Build history of the part. All positions in model axes, mm. A direction names the side the tool comes from. Give positions to 0.01 mm unless a question says otherwise; leave off trailing zeros. Write each loop counter-clockwise with the first axis right and the second up, starting at its lowest first coordinate (ties: lowest second). Pieces come first, ordered by that corner, then holes.
from build123d import *

# Parameters (mm, degrees)
BASEHEAD_DEPTH = 4
SKETCH5_R      = 3
BASEBODY_DEPTH = 30
CHAMFER1_SIZE  = 0.3
SCALE_1_SCALE  = 0.25


with BuildPart() as part:
    # Sketch2 → BaseHead (new body)
    with BuildSketch(Plane(origin=(0, 0, 0), x_dir=(0, 0, -1), z_dir=(1, 0, 0))):
        Polygon((0, -5.773502692), (5, -2.886751346), (5, 2.886751346), (0, 5.773502692), (-5, 2.886751346), (-5, -2.886751346), align=None)
    extrude(amount=BASEHEAD_DEPTH)

    # Sketch3 → BearingFace (revolve, cut)
    with BuildSketch(Plane.XY, mode=Mode.PRIVATE) as bearingface_sk:
        Polygon((4, 5.773502692), (4, 4.37), (3.5, 4.87), (3.5, 5.773502692), align=None)
    revolve(bearingface_sk.sketch.rotate(Axis((-0.957090588, 0, 0), (1, 0, 0)), 90), axis=Axis((-0.957090588, 0, 0), (1, 0, 0)), mode=Mode.SUBTRACT)

    # Sketch4 → HeadChamfer (revolve, cut)
    with BuildSketch(Plane.XY):
        Polygon((0, 5.773502692), (0.281531956, 5.773502692), (0, 5), align=None)
    revolve(axis=Axis((-0.493528746, 0, 0), (1, 0, 0)), mode=Mode.SUBTRACT)

    # Sketch5 → BaseBody (add)
    with BuildSketch(Plane(origin=(4, 0, 0), x_dir=(0, 0, -1), z_dir=(1, 0, 0))):
        with Locations(Location((0, 0, 0), (0, 0, 180))):
            Circle(SKETCH5_R)
    extrude(amount=BASEBODY_DEPTH)

    # Chamfer1
    chamfer1_edges = [part.edges().sort_by_distance(p)[0] for p in [
        (34, 0, -3),
    ]]
    chamfer(chamfer1_edges, length=CHAMFER1_SIZE)


with BuildPart() as part_1:
    # 缩放比例1: scaled about (0, 0, 0)
    add(part.part.scale(SCALE_1_SCALE))


solid = part_1.part
(1) Drop a flat-ended pin along its axis: pin 1 (1.5 mm diameter, centred on x = 3, z = 0, fed in from -Y). Give the stop position or say it passes through.
(2) Saw through at B-B, the plane x = 5. List the corners of the cut face in (y, z).
(3) Saw through at A-A, the plane x = 0.5. List the corners of the cut face in (y, z).
(4) Probe line 1 (Z direction, x = 4.5, y = 0.2); line 2 (X direction, y = -0.2, z = -0.9). List the from-to ranges inside material, lowest first.
(5) 3-axis set-ups, long thin cutter, end or side, ignore diameter. For faces 1 (the face through (4.661, -0.225, 0.715)), 2 (the face through (0.4, 0, 1.25)): which of +Z, -Z, +X, -X, +Y, -Y reach the whole face in a straight line?
Computed values:
1. pin 1: stops at y = -0.75
2. outline: circle Ø1.5 at (0, 0)
3. outline: (-1.44, 0) - (-0.72, -1.25) - (0.72, -1.25) - (1.44, 0) - (0.72, 1.25) - (-0.72, 1.25) - close
4. line 1: z = -0.72 to 0.72
4. line 2: x = 0 to 1
5. face 1: +X
5. face 2: +Z, +X, -X, +Y, -Y
